```python
from build123d import *

# Parameters (mm, degrees)
F0_W     = 18
F0_H     = 46
F1_DEPTH = 9
F2_W     = 38
F2_H     = 4
F3_DEPTH = 18.001
F4_R     = 2


with BuildPart() as f1:
    # F0 (on Top) → F1 (new body)
    with BuildSketch(Plane.XY):
        Rectangle(F0_W, F0_H)
    extrude(amount=F1_DEPTH)

    # F2 (on face) → F3 (cut, through all)
    with BuildSketch(Plane.YZ.offset(9)):
        with Locations((0, 4.5)):
            Rectangle(F2_W, F2_H)
    extrude(amount=-F3_DEPTH, mode=Mode.SUBTRACT)

    # F4
    f4_edges = [f1.edges().sort_by_distance(p)[0] for p in [
        (0, -23, 9),
        (0, -23, 0),
        (0, 23, 9),
        (0, 23, 0),
    ]]
    fillet(f4_edges, radius=F4_R)


solid = f1.part
```
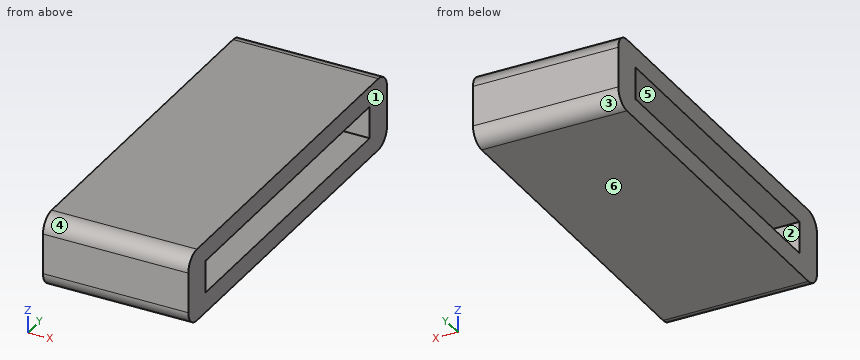
Here's how the part is built. I have some questions about the finished solid (model axes, mm). Face numbers are marked on the shaded views. A direction names the side the tool comes from. Coordinates: 2 decimals unless noted, no trailing zeros. Loops run counter-clockwise (first coordinate to the right, second up) from the corner with the lowest first, then second, coordinate; pieces in that order, holes last. Notation, with made-up numbers: M 87,-23 L 137,-23 A22 ccw 137,3 Z; hole C 59.25,49.5 d10. An arc over 180 degrees is marked long. One line per item, written item: value.
1. Please list where these lines run through material, in increasing order: probe 1 along Z at (x, y) = (2, 18); probe 2 along Y at (x, z) = (-1.5, 3.75); probe 3 along Y at (x, z) = (-7.5, 0.5).
Geometry says:
probe 1: z = 0 to 2.5, 6.5 to 9
probe 2: y = -23 to -19, 19 to 23
probe 3: y = -22.32 to 22.32
2. Imagine slicing it at B-B (y = 1.5). List the corners of the cut face in (x, z) for me, and give its area (3 significant figures).
Geometry says:
outline: M -9,0 L 9,0 L 9,2.5 L -9,2.5 Z; M -9,6.5 L 9,6.5 L 9,9 L -9,9 Z
area: 90.0 mm2
3. Imagine slicing it at A-A (z = 5.25). List the corners of the cut face in (x, y) for me, and give its area (3 significant figures).
Geometry says:
outline: M -9,-23 L 9,-23 L 9,-19 L -9,-19 Z; M -9,19 L 9,19 L 9,23 L -9,23 Z
area: 144 mm2
4. Imagine slicing it at C-C (x = 3.5). List the corners of the cut face in (y, z) for me.
Geometry says:
outline: M -23,2 A2 ccw -21,0 L 21,0 A2 ccw 23,2 L 23,7 A2 ccw 21,9 L -21,9 A2 ccw -23,7 Z; hole M -19,2.5 L 19,2.5 L 19,6.5 L -19,6.5 Z
5. On a 3-axis mill with a long thin cutter (end or side, diameter ignored), from which of +Z, -Z, +X, -X, +Y, -Y can I reach the whole of each face in a straight line? I mean the marked faces 5 and 6. Say none if no direction works.
Geometry says:
face 5: +X, -X
face 6: -Z, +X, -X, +Y, -Y
6. Thinking about a two-plate mould opening in Z: for the marked faces 1, 2, 3 and 4, which applies, +Z half, -Z half, draft (parallel to the pull), parting line (faces both ways), or undercut?
Geometry says:
face 1: draft
face 2: undercut
face 3: -Z half
face 4: +Z half
